from build123d import *

# Parameters (mm, degrees)
SKETCH_1_R             = 16.5
SKETCH_1_R_2           = 2.1
SM_BASE_FLANGE_1_DEPTH = 4
FILLET_1_R             = 5
SKETCH_2_R             = 2
CUT_EXTRUDE_1_DEPTH    = 10


# Sheet-metal steps are written as plain solids
with BuildPart() as part:
    # Sketch 1 → Базовая кромка1 (new body)
    with BuildSketch(Plane(origin=(0, 0, 0), x_dir=(1, 0, 0), z_dir=(0, 1, 0))):
        with BuildLine():
            Line((-162.69465723, 365.418183057), (-138.290458646, 310.605455598))
            ThreePointArc((-138.290458646, 310.605455598), (0, 340), (138.290458646, 310.605455598))
            Line((138.290458646, 310.605455598), (162.69465723, 365.418183057))
            ThreePointArc((162.69465723, 365.418183057), (0, 400), (-162.69465723, 365.418183057))
        make_face()
        with Locations(Location((30.960802033, 368.702357922, 0), (0, 0, 270))):
            Circle(SKETCH_1_R, mode=Mode.SUBTRACT)
        with Locations(Location((-30.960802033, 368.702357922, 0), (0, 0, 270))):
            Circle(SKETCH_1_R, mode=Mode.SUBTRACT)
        with Locations(Location((92.015258251, 358.375769618, 0), (0, 0, 270))):
            Circle(SKETCH_1_R, mode=Mode.SUBTRACT)
        with Locations(Location((-92.015258251, 358.375769618, 0), (0, 0, 270))):
            Circle(SKETCH_1_R, mode=Mode.SUBTRACT)
        with Locations(Location((0, 350, 0), (0, 0, 270))):
            Circle(SKETCH_1_R_2, mode=Mode.SUBTRACT)
        with Locations(Location((0, 390, 0), (0, 0, 270))):
            Circle(SKETCH_1_R_2, mode=Mode.SUBTRACT)
    extrude(amount=-SM_BASE_FLANGE_1_DEPTH)

    # Скругление1
    fillet_1_edges = [part.edges().sort_by_distance(p)[0] for p in [
        (-138.290458646, -2, -310.605455598),
        (-162.69465723, -2, -365.418183057),
        (162.69465723, -2, -365.418183057),
        (138.290458646, -2, -310.605455598),
    ]]
    fillet(fillet_1_edges, radius=FILLET_1_R)

    # Эскиз2 → Вырез-Вытянуть1 (cut)
    with BuildSketch(Plane(origin=(0, 0, 0), x_dir=(1, 0, 0), z_dir=(0, 1, 0))):
        with Locations(Location((156.080374798, 362.85522816, 0), (0, 0, 270))):
            Circle(SKETCH_2_R)
        with Locations(Location((135.741676964, 317.173764891, 0), (0, 0, 270))):
            Circle(SKETCH_2_R)
        with Locations(Location((-135.741676964, 317.173764891, 0), (0, 0, 270))):
            Circle(SKETCH_2_R)
        with Locations(Location((-156.080374798, 362.85522816, 0), (0, 0, 270))):
            Circle(SKETCH_2_R)
    extrude(amount=-CUT_EXTRUDE_1_DEPTH, mode=Mode.SUBTRACT)


solid = part.part
Geometry check sheet. Reference: the model listing, model coordinates, mm. Coordinates: 2 decimals unless noted, no trailing zeros. Write each loop counter-clockwise with the first axis right and the second up, starting at its lowest first coordinate (ties: lowest second). Pieces come first, ordered by that corner, then holes. Notation, with made-up numbers: (0, 49) -> (51, 49) arc R7 ccw to (51, 62) -> close; hole circle Ø9 at (-39, 39.5). An arc over 180 degrees is marked (long way). One line per question, with ' | ' between items.
1. Cross-section at C-C on x = 6.5. Record the cut outline in (y, z).
Answers:
outline: (-4, -399.95) -> (0, -399.95) -> (0, -339.94) -> (-4, -339.94) -> close
2. Cross-section at A-A on x = 78.5. Record the cut outline in (y, z).
Answers:
outline: (-4, -392.22) -> (0, -392.22) -> (0, -367.84) -> (-4, -367.84) -> close; (-4, -348.91) -> (0, -348.91) -> (0, -330.81) -> (-4, -330.81) -> close
3. Thickness scan on probe 1 along X at (y, z) = (-1.95, -350); probe 2 along X at (y, z) = (-3.8, -346.5); probe 3 along X at (y, z) = (-0.9, -349). Record the ranges inside material, lowest first. Write a range as from..to.
Answers:
probe 1: x = -155.83..-106.23, -77.8..-2.1, 2.1..77.8, 106.23..155.83 | probe 2: x = -154.27..-103.47, -80.56..80.56, 103.47..154.27 | probe 3: x = -155.38..-105.59, -78.44..-1.85, 1.85..78.44, 105.59..155.38
4. Cross-section at B-B on z = -323. Record the cut outline in (x, y), and give its area (3 significant figures).
Answers:
outline: (-143.81, -4) -> (-106.16, -4) -> (-106.16, 0) -> (-143.81, 0) -> close; (106.16, -4) -> (143.81, -4) -> (143.81, 0) -> (106.16, 0) -> close | area: 301 mm²
5. Cross-section at D-D on x = -59. Record the cut outline in (y, z), and give its area (3 significant figures).
Answers:
outline: (-4, -395.62) -> (0, -395.62) -> (0, -334.84) -> (-4, -334.84) -> close | area: 243 mm²
6. Depth check by flat-ended pin: pin 1 Ø4 at (x, z) = (0, -350) entering from +Y. Enter the tip coordinate at first touch or a pass-through.
Answers:
pin 1: passes through
7. Draft check along X on faces 1 (the flat face through (-2, 0, -357)), 2 (the cylindrical face through (-87.059, -1.972, -342.638)), 3 (the cylindrical face through (96.971, -1.972, -342.638)), 4 (the flat face through (150.336, -1.972, -337.661)). Enter one of: +X half, -X half, draft (parallel to the pull), parting line (faces both ways), or undercut.
Answers:
face 1: draft | face 2: undercut | face 3: undercut | face 4: +X half
